Read the model definition and answer for the solid it produces. Units are mm, in the model's axes. A direction names the side the tool comes from. Coordinates: 2 decimals unless noted, no trailing zeros. Order: outer loops, then holes, each group sorted by start corner. A loop starts at its lowest first (then second) coordinate and runs counter-clockwise, first axis right, second up. Notation, with made-up numbers: (-8.5, 17) -> (12.5, 17) arc R20 ccw to (12.5, 50) -> close; hole circle Ø6 at (18.25, 15). An arc over 180 degrees is marked (long way). Return JSON: item names as keys, results as strings. Group by question number.
```python
from build123d import *

# Parameters (mm, degrees)
SKETCH1_W           = 229
SKETCH1_H           = 26
BOSS_EXTRUDE1_DEPTH = 3
SKETCH2_W           = 229
SKETCH2_H           = 3
BOSS_EXTRUDE2_DEPTH = 24
SKETCH3_W           = 31
SKETCH3_H           = 4
CUT_EXTRUDE1_DEPTH  = 24


with BuildPart() as part:
    # Sketch1 → Boss-Extrude1 (new body)
    with BuildSketch(Plane(origin=(0, 0, 0), x_dir=(1, 0, 0), z_dir=(0, 1, 0))):
        with Locations((-114.5, -13)):
            Rectangle(SKETCH1_W, SKETCH1_H)
    extrude(amount=BOSS_EXTRUDE1_DEPTH)

    # Sketch2 → Boss-Extrude2 (add)
    with BuildSketch(Plane(origin=(0, 3, 0), x_dir=(1, 0, 0), z_dir=(0, 1, 0))):
        with Locations((-114.5, -1.5)):
            Rectangle(SKETCH2_W, SKETCH2_H)
    extrude(amount=BOSS_EXTRUDE2_DEPTH)

    # Sketch3 → Cut-Extrude1 (cut)
    with BuildSketch(Plane.XY.offset(3)):
        with Locations((-213.5, 5)):
            Rectangle(SKETCH3_W, SKETCH3_H)
        with Locations((-15.5, 5)):
            Rectangle(SKETCH3_W, SKETCH3_H)
    extrude(amount=-CUT_EXTRUDE1_DEPTH, mode=Mode.SUBTRACT)


solid = part.part
```
1. A straight line is drawn through the part: L1, parallel to Y at x = -101, z = 11. Find the intervals that lie inside material, in ascending order.
2. Given pin 1 (4 mm diameter, centred on x = -42.5, y = 9, fed in from +Z); pin 2 (2.5 mm diameter, centred on y = 4.5, z = 1.5, fed in from -X); pin 3 (6 mm diameter, centred on x = -118.5, z = 19.5, fed in from +Y), each flat-ended and moving along its own axis, determine where each tip first touches the part or whether it passes through.
3. Find section B-B on z = 16.5. Determine the outline of the cut face in (x, y), and give its area (3 significant figures).
4. Find section A-A on x = -79. Determine the outline of the cut face in (y, z), and give its area (3 significant figures).
5. Which of the six approach directions +Z, -Z, +X, -X, +Y, -Y give full straight-line access (tool end or side, diameter ignored) to faces 1 (the face through (-116, 0, 13)), 2 (the face through (-116, 15, 3))?
Result:
{
 "1": {"L1": "0 to 3"},
 "2": {"pin 1": "z = 3", "pin 2": "x = -198", "pin 3": "y = 3"},
 "3": {"outline": "(-229, 0) -> (0, 0) -> (0, 3) -> (-229, 3) -> close", "area": "687 mm^2"},
 "4": {"outline": "(0, 0) -> (27, 0) -> (27, 3) -> (3, 3) -> (3, 26) -> (0, 26) -> close", "area": "150 mm^2"},
 "5": {"face 1": "+Z, -Z, +X, -X, -Y", "face 2": "+Z, +X, -X, +Y"}
}
